```python
from build123d import *

# Parameters (mm, degrees)
BOSS_EXTRUDE1_DEPTH        = 6.5786
F_97_0_25_DIAMETER_HOLE1_D = 6.35


with BuildPart() as part:
    # Sketch2 → Boss-Extrude1 (new body)
    with BuildSketch(Plane.XY):
        with BuildLine():
            Line((-16.66875, -15.734319794), (-16.66875, -39.617329943))
            Line((-16.66875, -39.617329943), (-16.66875, -49.389319794))
            Line((-16.66875, -49.389319794), (-16.66875, -53.212823447))
            Line((-16.66875, -53.212823447), (-50.00625, -53.212823447))
            Line((-50.00625, -53.212823447), (-50.00625, 22.987176553))
            Line((-50.00625, 22.987176553), (-11.90625, 22.987176553))
            Line((-11.90625, 22.987176553), (-11.90625, 13.589176553))
            ThreePointArc((-11.90625, 13.589176553), (-20.281897601, 4.630319933), (-18.935193267, -7.559797873))
            ThreePointArc((-18.935193267, -7.559797873), (-17.24585042, -11.492870345), (-16.66875, -15.734319794))
        make_face()
    extrude(amount=BOSS_EXTRUDE1_DEPTH)

    # #97 (0.25) Diameter Hole1 (through all)
    with Locations(Plane(origin=(-37.30625, 10.287176553, 6.5786), x_dir=(1, 0, 0), z_dir=(0, 0, 1))):
        with Locations((0, 0), (0, -50.8)):
            Hole(F_97_0_25_DIAMETER_HOLE1_D / 2)


solid = part.part
```
Geometry check sheet. Reference: the model listing, model coordinates, mm. A direction names the side the tool comes from. Give positions to 0.01 mm unless a question says otherwise; leave off trailing zeros. Order: outer loops, then holes, each group sorted by start corner. A loop starts at its lowest first (then second) coordinate and runs counter-clockwise, first axis right, second up. Notation, with made-up numbers: (-2.5, 20.25) - (40.5, 20.25) arc R29 cw to (40.5, 49.25) - close; hole circle Ø1 at (-32, -15.75). An arc over 180 degrees is marked (long way). Answer in a Markdown table with one row per item. Add a question column.
Q1. Cross-section at A-A, the plane y = -39.5. Enter the section's corners in (x, z).
Q2. Tool access check on faces 5 (the flat face through (-31, -15, 0)), 6 (the flat face through (-16.669, -34, 3)), 7 (the cylindrical face through (-17.262, -11.435, 3.243)). Record the directions out of +Z, -Z, +X, -X, +Y, -Y that give a thin tool (end or side, any length) a straight path to the whole face; none if there is none.
Q3. Cross-section at C-C, the plane x = -37. Enter the section's corners in (y, z).
Q4. Material ranges on probe 1 along X at (y, z) = (-36, 2.25); probe 2 along X at (y, z) = (11, 6); probe 3 along X at (y, z) = (0.5, 0.5), recorded low to high. Write a range as from..to.
Q5. Cross-section at B-B, the plane x = -18. Enter the section's corners in (y, z), then the cut area to 3 significant figures.
Q6. Mould release check, pull along Y, two halves, no side actions. Record for faces 1 (the flat face through (-31, 22.987, 3)), 2 (the cylindrical face through (-34.966, 12.433, 3.243)), 3 (the flat face through (-50.006, -16, 3)), 4 (the flat face through (-33, -53.213, 3)): pulls with the +Y half, pulls with the -Y half, needs draft (parallel to the pull), parting line crosses it, or undercut.
Q7. Cross-section at D-D, the plane z = 0.75. Enter the section's corners in (x, y) (3 decimals).
Check values:
| question | item | result |
|---|---|---|
| 1 | outline | (-50.01, 0) - (-40.32, 0) - (-40.32, 6.58) - (-50.01, 6.58) - close; (-34.3, 0) - (-16.67, 0) - (-16.67, 6.58) - (-34.3, 6.58) - close |
| 2 | face 5 | -Z, +X, -X, +Y, -Y |
| 2 | face 6 | +Z, -Z, +X, -Y |
| 2 | face 7 | +Z, -Z, +X |
| 3 | outline | (-53.21, 0) - (-43.67, 0) - (-43.67, 6.58) - (-53.21, 6.58) - close; (-37.35, 0) - (7.13, 0) - (7.13, 6.58) - (-37.35, 6.58) - close; (13.45, 0) - (22.99, 0) - (22.99, 6.58) - (13.45, 6.58) - close |
| 4 | probe 1 | x = -50.01..-16.67 |
| 4 | probe 2 | x = -50.01..-40.4, -34.21..-16.07 |
| 4 | probe 3 | x = -50.01..-21.02 |
| 5 | outline | (-53.21, 0) - (-9.37, 0) - (-9.37, 6.58) - (-53.21, 6.58) - close; (8.93, 0) - (22.99, 0) - (22.99, 6.58) - (8.93, 6.58) - close |
| 5 | area | 381 mm^2 |
| 6 | face 1 | pulls with the +Y half |
| 6 | face 2 | undercut |
| 6 | face 3 | needs draft |
| 6 | face 4 | pulls with the -Y half |
| 7 | outline | (-50.006, -53.213) - (-16.669, -53.213) - (-16.669, -15.734) arc R15.875 ccw to (-18.935, -7.56) arc R14.681 cw to (-11.906, 13.589) - (-11.906, 22.987) - (-50.006, 22.987) - close; hole circle Ø6.35 at (-37.306, -40.513); hole circle Ø6.35 at (-37.306, 10.287) |
